Could you check a few things on this model? Use its own coordinates, in mm. Give positions to 0.01 mm unless a question says otherwise; leave off trailing zeros. Order: outer loops, then holes, each group sorted by start corner. A loop starts at its lowest first (then second) coordinate and runs counter-clockwise, first axis right, second up. Notation, with made-up numbers: M -15,13 L 32,13 A10 cw 32,19 Z; hole C 26,42 d3. An arc over 180 degrees is marked long. Use a Markdown table: item, result. Add a question column.
```python
from build123d import *

# Parameters (mm, degrees)
F2_ANGLE = 180


with BuildPart() as f2:
    # F0 (on Front) → F2 (revolve)
    with BuildSketch(Plane.XZ):
        Polygon((42.950819, 0), (-48.825024, 0), (-25.797102, -39.497256), (19.922898, -39.497256), align=None)
        Polygon((-25.797102, 39.497256), (-48.825024, 0), (42.950819, 0), (19.922898, 39.497256), align=None)
    revolve(axis=Axis((-2.501527, 0, 64.897256), (1, 0, 0)), revolution_arc=F2_ANGLE)


solid = f2.part
```
1) Suppose I cut it at B-B on x = -31.5. Please give me the cut outline in (y, z), and give its area (3 significant figures).
2) We'd pull the mould along Z, two halves only. Please class faces 1 (the face through (-2.62, 104.37, 62.6)), 2 (the face through (-29.796, 32.252, 64.188)), 3 (the face through (-4, 0, 129)): pulls with the +Z half, pulls with the -Z half, needs draft (parallel to the pull), parting line crosses it, or undercut.
3) For pin 1 (4 mm diameter, centred on x = -9.5, y = 87.5, fed in from +Z); pin 2 (1.5 mm diameter, centred on x = 2.5, y = 41, fed in from +Z); pin 3 (1.5 mm diameter, centred on x = -10.5, z = 84.5, fed in from -Y), each with a flat end and sliding along its axis, tell me the tip position at first contact or that it passes through.
4) Please list where these lines run through material, in increasing order: line 1 (Z direction, x = 1.5, y = 22.5); line 2 (Z direction, x = 37.5, y = 31.5); line 3 (Y direction, x = 20, z = 133.5). Write a range as from..to.
5) Suppose I cut it at A-A on x = -5. Please give me the cut outline in (y, z).
Values found:
| question | item | result |
|---|---|---|
| 1 | outline | M 0,-29.72 A94.61 ccw 0,159.51 L 0,100.08 A35.18 cw 0,29.72 Z |
| 1 | area | 12,100 mm^2 |
| 2 | face 1 | parting line crosses it |
| 2 | face 2 | undercut |
| 2 | face 3 | needs draft |
| 3 | pin 1 | stops at z = 124.8 |
| 3 | pin 2 | stops at z = 161.22 |
| 3 | pin 3 | stops at y = 15.2 |
| 4 | line 1 | z = -37.04..53.11, 76.68..166.84 |
| 4 | line 2 | z = -2.34..19.14, 110.65..132.13 |
| 4 | line 3 | y = 0..78.51 |
| 5 | outline | M 0,-39.5 A104.39 ccw 0,169.29 L 0,90.3 A25.4 cw 0,39.5 Z |
